```python
from build123d import *

# Parameters (mm, degrees)
SKETCH1_W               = 228.6
SKETCH1_H               = 25.4
BOSS_EXTRUDE1_DEPTH     = 1.016
BOSS_EXTRUDE2_START     = -25.4
BOSS_EXTRUDE2_OUTLINE_R = 3.175
BOSS_EXTRUDE2_DEPTH     = 25.4
CUT_EXTRUDE2_DEPTH      = 240.548137597


# Read off the part's stored shape, not the designer's step: Boss-Extrude2
with BuildPart() as part:
    # Sketch1 → Boss-Extrude1 (new body)
    with BuildSketch(Plane(origin=(0, 0, 0), x_dir=(1, 0, 0), z_dir=(0, 1, 0))):
        with Locations((114.3, 0)):
            Rectangle(SKETCH1_W, SKETCH1_H)
    extrude(amount=BOSS_EXTRUDE1_DEPTH)

    # Boss-Extrude2 outline → Boss-Extrude2 (add)
    with BuildSketch(Plane(origin=(0, 0, -12.7), x_dir=(-1, 0, 0), z_dir=(0, 0, -1)).offset(BOSS_EXTRUDE2_START)):
        with BuildLine():
            ThreePointArc((-229.658333333, 7.184418707), (-225.486151946, 14.050397837), (-231.381237899, 19.509035812))
            add(Edge.make_bspline(
                [(-231.381237899, 19.509035812), (-236.227087861, 19.810105296), (-241.340763982, 15.106028372), (-239.097965647, 8.031629833), (-236.573095563, 0), (-228.6, 0)],
                knots=[0, 0, 0, 0, 0, 0, 1, 1, 1, 1, 1, 1], degree=5))
            Line((-228.6, 0), (-228.6, 1.016))
            ThreePointArc((-228.6, 1.016), (-231.729275427, 3.654101218), (-229.658333333, 7.184418707))
        make_face()
        with Locations((-231.775, 13.171256121)):
            Circle(BOSS_EXTRUDE2_OUTLINE_R, mode=Mode.SUBTRACT)
    extrude(amount=BOSS_EXTRUDE2_DEPTH)

    # Sketch3 → Cut-Extrude2 (cut, through all)
    with BuildSketch(Plane.XZ):
        Polygon((226.576403153, 12.7), (238.413448409, 5.865878735), (238.413448409, 12.7), align=None)
        Polygon((226.576403153, -12.7), (238.413448409, -5.865878735), (238.413448409, -12.7), align=None)
    extrude(amount=-CUT_EXTRUDE2_DEPTH, mode=Mode.SUBTRACT)


solid = part.part
```
Input: part model. Units: mm. Frame: model coordinates. Round coordinates to 2 decimals unless told otherwise and drop trailing zeros. Loops run counter-clockwise (first coordinate to the right, second up) from the corner with the lowest first, then second, coordinate; pieces in that order, holes last. Notation, with made-up numbers: (-30, 18.25) -> (16, 18.25) arc R17 ccw to (16, 39.25) -> close; hole circle Ø1 at (-6, 87). An arc over 180 degrees is marked (long way). Use one line per item in the form item = value. Start each with the question number.
Item 1: Section query A-A on x = 154. Return the cut outline in (y, z), then the cut area to 3 significant figures.
Item 2: Material intervals for L1, parallel to Y at x = 26.5, z = 7.25; L2, parallel to X at y = 13.75, z = -6.75; L3, parallel to X at y = 10.75, z = 4, sorted ascending. Write a range as from..to.
Item 3: Contact query for flat-ended pins moving along their axis: pin 1 Ø4 at (x, z) = (181.5, 1.5) entering from +Y; pin 2 Ø5 at (y, z) = (8, 4.5) entering from -X; pin 3 Ø5.5 at (x, y) = (231.78, 13.17) entering from +Z; pin 4 Ø8 at (y, z) = (17.5, 5.5) entering from +X. Output: stop coordinate, or through.
Item 4: Mould query, pull axis Y, two halves, no side actions, for faces 1 (the face through (231.718, 3.593, 0.161)), 2 (the face through (113, 0, 0)), 3 (the face through (232.41, 9.63, 9.33)). Classes: pulls with the +Y half, pulls with the -Y half, needs draft (parallel to the pull), parting line crosses it, or undercut.
Ans:
q1.outline = (0, -12.7) -> (1.02, -12.7) -> (1.02, 12.7) -> (0, 12.7) -> close
q1.area = 25.8 mm^2
q2.L1 = 0..1.02
q2.L2 = 225.45..228.65, 234.9..236.88
q2.L3 = 225.9..229.72, 233.83..238.37
q3.pin_1 = 1.02
q3.pin_2 = 226.01
q3.pin_3 = through
q3.pin_4 = 238.27
q4.face_1 = undercut
q4.face_2 = pulls with the -Y half
q4.face_3 = needs draft
